```python
from build123d import *

# Parameters (mm, degrees)
SKETCH_1_W               = 36
SKETCH_1_H               = 32
EXTRUDE_1_DEPTH          = 5
SKETCH_4_W               = 33
SKETCH_4_H               = 12
CUT_EXTRUDE_2_DEPTH      = 2
SKETCH_8_R               = 1
CUT_EXTRUDE_6_DEPTH      = 3
CUT_EXTRUDE_3_DEPTH      = 25.269322199
CUT_EXTRUDE_3_DEPTH_BACK = 3
SKETCH_5_W               = 23.5
SKETCH_5_H               = 12
SKETCH_11_W              = 15
SKETCH_11_H              = 5
EXTRUDE_3_DEPTH          = 30
CUT_EXTRUDE_8_REACH      = 49.413
SKETCH_12_R              = 5
CUT_EXTRUDE_9_REACH      = 40.471
SKETCH_13_R              = 1.05


with BuildPart() as part:
    # 草图1 → 凸台-拉伸1 (new body)
    with BuildSketch(Plane(origin=(0, 0, 0), x_dir=(1, 0, 0), z_dir=(0, 1, 0))):
        Rectangle(SKETCH_1_W, SKETCH_1_H)
    extrude(amount=EXTRUDE_1_DEPTH)

    # 草图4 → 切除-拉伸2 (cut)
    with BuildSketch(Plane.XZ):
        Rectangle(SKETCH_4_W, SKETCH_4_H)
    extrude(amount=-CUT_EXTRUDE_2_DEPTH, mode=Mode.SUBTRACT)

    # 草图8 → 切除-拉伸6 (cut)
    with BuildSketch(Plane.XZ.offset(-2)):
        with Locations(Location((14, 0, 0), (0, 0, 270))):
            Circle(SKETCH_8_R)
        with Locations(Location((-14, 0, 0), (0, 0, 270))):
            Circle(SKETCH_8_R)
    extrude(amount=-CUT_EXTRUDE_6_DEPTH, mode=Mode.SUBTRACT)

    # 草图5 → 切除-拉伸3 (cut, two sides: drawn at the far end of the back side and taken through both)
    with BuildSketch(Plane.XZ.offset(-2).offset(-CUT_EXTRUDE_3_DEPTH_BACK)):
        Rectangle(SKETCH_5_W, SKETCH_5_H)
    extrude(amount=CUT_EXTRUDE_3_DEPTH + CUT_EXTRUDE_3_DEPTH_BACK, mode=Mode.SUBTRACT)

    # 草图11 → 凸台-拉伸3 (add)
    with BuildSketch(Plane.XZ):
        with Locations((0, 13.5)):
            Rectangle(SKETCH_11_W, SKETCH_11_H)
        with Locations((0, -13.5)):
            Rectangle(SKETCH_11_W, SKETCH_11_H)
    extrude(amount=EXTRUDE_3_DEPTH)

    # 切除-拉伸8: up to this face of the body (flat: up to its plane)
    cut_extrude_8_end = Plane(part.part.faces().sort_by_distance((0, -10, 16))[0])
    # 草图12 → 切除-拉伸8 (cut, up to the picked face)
    with BuildSketch(Plane(origin=(0, 0, -16), x_dir=(-1, 0, 0), z_dir=(0, 0, -1)), mode=Mode.PRIVATE) as cut_extrude_8_sk1:
        with Locations((0, -23)):
            Circle(SKETCH_12_R)
    cut_extrude_8_tool1 = split(extrude(cut_extrude_8_sk1.sketch, amount=-CUT_EXTRUDE_8_REACH, mode=Mode.PRIVATE), bisect_by=cut_extrude_8_end, keep=Keep.BOTH, mode=Mode.PRIVATE)
    add(cut_extrude_8_tool1.solids().sort_by(Axis((0, -23, -16), (0, 0, 1)))[0], mode=Mode.SUBTRACT)

    # 草图13 → 切除-拉伸9 (cut, up to next)
    with BuildSketch(Plane.XZ, mode=Mode.PRIVATE) as cut_extrude_9_sk1:
        with Locations(Location((-12, 14, 0), (0, 0, 270))):
            Circle(SKETCH_13_R)
    cut_extrude_9_tool1 = extrude(cut_extrude_9_sk1.sketch, amount=-CUT_EXTRUDE_9_REACH, mode=Mode.PRIVATE) & part.part
    # 草图13 → 切除-拉伸9 (cut, up to next)
    with BuildSketch(Plane.XZ, mode=Mode.PRIVATE) as cut_extrude_9_sk2:
        with Locations(Location((12, 14, 0), (0, 0, 90))):
            Circle(SKETCH_13_R)
    cut_extrude_9_tool2 = extrude(cut_extrude_9_sk2.sketch, amount=-CUT_EXTRUDE_9_REACH, mode=Mode.PRIVATE) & part.part
    # 草图13 → 切除-拉伸9 (cut, up to next)
    with BuildSketch(Plane.XZ, mode=Mode.PRIVATE) as cut_extrude_9_sk3:
        with Locations(Location((12, -14, 0), (0, 0, 270))):
            Circle(SKETCH_13_R)
    cut_extrude_9_tool3 = extrude(cut_extrude_9_sk3.sketch, amount=-CUT_EXTRUDE_9_REACH, mode=Mode.PRIVATE) & part.part
    # 草图13 → 切除-拉伸9 (cut, up to next)
    with BuildSketch(Plane.XZ, mode=Mode.PRIVATE) as cut_extrude_9_sk4:
        with Locations(Location((-12, -14, 0), (0, 0, 90))):
            Circle(SKETCH_13_R)
    cut_extrude_9_tool4 = extrude(cut_extrude_9_sk4.sketch, amount=-CUT_EXTRUDE_9_REACH, mode=Mode.PRIVATE) & part.part
    add(cut_extrude_9_tool1.solids().sort_by_distance((-12, 0, 14))[0], mode=Mode.SUBTRACT)
    add(cut_extrude_9_tool2.solids().sort_by_distance((12, 0, 14))[0], mode=Mode.SUBTRACT)
    add(cut_extrude_9_tool3.solids().sort_by_distance((12, 0, -14))[0], mode=Mode.SUBTRACT)
    add(cut_extrude_9_tool4.solids().sort_by_distance((-12, 0, -14))[0], mode=Mode.SUBTRACT)


solid = part.part
```
Verification items for the finished model (mm, model axes). A direction names the side the tool comes from. Give positions to 0.01 mm unless a question says otherwise; leave off trailing zeros. Order: outer loops, then holes, each group sorted by start corner. A loop starts at its lowest first (then second) coordinate and runs counter-clockwise, first axis right, second up. Notation, with made-up numbers: (66.25, 74.25) -> (119.25, 74.25) arc R13 cw to (119.25, 80.25) -> close; hole circle Ø3 at (76.5, -29.5). An arc over 180 degrees is marked (long way). One line per item, written item: value.
(1) Tool access check on faces 1 (the face through (0, -15, -11)), 2 (the face through (7.5, -15, 13)), 3 (the face through (-16.5, 1, 0)), 4 (the face through (-7.5, -15, 13)), 5 (the face through (-11.75, 4, 0)). Record the directions out of +Z, -Z, +X, -X, +Y, -Y that give a thin tool (end or side, any length) a straight path to the whole face; none if there is none.
Final values:
face 1: +X, -X, -Y
face 2: +Z, -Z, +X, -Y
face 3: -Y
face 4: +Z, -Z, -X, -Y
face 5: +Y, -Y
(2) Gauge pin test, flat ends, axial feed: pin 1 (6 mm diameter, centred on x = 12, y = -5.5, fed in from -Z); pin 2 (3 mm diameter, centred on y = -7.5, z = -12, fed in from +X); pin 3 (10 mm diameter, centred on x = 1, y = -20, fed in from +Z); pin 4 (1.5 mm diameter, centred on x = 9, z = 11, fed in from -Y). Record the tip position at first contact, or that the pin passes through.
Final values:
pin 1: through
pin 2: x = 7.5
pin 3: z = 16
pin 4: y = 0
(3) Sectioned sample at C-C on x = 0. Record the cut outline in (y, z), then the cut area to 3 significant figures.
Final values:
outline: (-30, -16) -> (-28, -16) -> (-28, -11) -> (-30, -11) -> close; (-30, 11) -> (-28, 11) -> (-28, 16) -> (-30, 16) -> close; (-18, -16) -> (5, -16) -> (5, -6) -> (0, -6) -> (0, -11) -> (-18, -11) -> close; (-18, 11) -> (0, 11) -> (0, 6) -> (5, 6) -> (5, 16) -> (-18, 16) -> close
area: 300 mm^2
(4) Sectioned sample at D-D on y = -26. Record the cut outline in (x, z).
Final values:
outline: (-7.5, -16) -> (-4, -16) -> (-4, -11) -> (-7.5, -11) -> close; (-7.5, 11) -> (-4, 11) -> (-4, 16) -> (-7.5, 16) -> close; (4, -16) -> (7.5, -16) -> (7.5, -11) -> (4, -11) -> close; (4, 11) -> (7.5, 11) -> (7.5, 16) -> (4, 16) -> close
(5) Scan lines: line 1 along X through (y, z) = (3.15, -14); line 2 along Y through (x, z) = (0, -13); line 3 along Z through (x, y) = (1, -8). Record each from-to range of solid material in increasing order. Write a range as [from, to].
Final values:
line 1: [-18, -13.05], [-10.95, 10.95], [13.05, 18]
line 2: [-30, -28], [-18, 5]
line 3: [-16, -11], [11, 16]
(6) Sectioned sample at A-A on z = -14. Record the cut outline in (x, y), then the cut area to 3 significant figures.
Final values:
outline: (-18, 0) -> (-13.05, 0) -> (-13.05, 5) -> (-18, 5) -> close; (-10.95, 0) -> (-7.5, 0) -> (-7.5, -30) -> (7.5, -30) -> (7.5, 0) -> (10.95, 0) -> (10.95, 5) -> (-10.95, 5) -> close; (13.05, 0) -> (18, 0) -> (18, 5) -> (13.05, 5) -> close; hole circle Ø10 at (0, -23)
area: 530 mm^2
(7) Draft check along Z on faces 6 (the face through (18, 2, 0)), 7 (the face through (-15.2, 2, 0.1)). Enter one of: pulls with the +Z half, pulls with the -Z half, needs draft (parallel to the pull), parting line crosses it, or undercut.
Final values:
face 6: needs draft
face 7: undercut
(8) Sectioned sample at B-B on z = 0. Record the cut outline in (x, y), then the cut area to 3 significant figures.
Final values:
outline: (-18, 0) -> (-16.5, 0) -> (-16.5, 2) -> (-15, 2) -> (-15, 5) -> (-18, 5) -> close; (-13, 2) -> (-11.75, 2) -> (-11.75, 5) -> (-13, 5) -> close; (11.75, 2) -> (13, 2) -> (13, 5) -> (11.75, 5) -> close; (15, 2) -> (16.5, 2) -> (16.5, 0) -> (18, 0) -> (18, 5) -> (15, 5) -> close
area: 31.5 mm^2
